Geometry check sheet. Reference: the model listing, model coordinates, mm. Face numbers are marked on the shaded views. A direction names the side the tool comes from. Give positions to 0.01 mm unless a question says otherwise; leave off trailing zeros. Write each loop counter-clockwise with the first axis right and the second up, starting at its lowest first coordinate (ties: lowest second). Pieces come first, ordered by that corner, then holes. Notation, with made-up numbers: (56, 2) - (61, 2) arc R18 cw to (61, 14) - close; hole circle Ø4 at (2, -21.5). An arc over 180 degrees is marked (long way). One line per question, with ' | ' between items. Start each with the question number.
Q1. Section check B-B on x = 0. Record the boundary of the cut face in (y, z).
Q2. Section check A-A on z = 0. Record the boundary of the cut face in (x, y), and give its area (3 significant figures).
Q3. Set-up check for the marked faces 4, 5 and 6: record each of +Z, -Z, +X, -X, +Y, -Y from which the full face is reachable in a straight line by a thin tool's end or side.
Q4. Thickness scan on L1, parallel to Y at x = 0.5, z = 0; L2, parallel to X at y = 53.5, z = 0; L3, parallel to Z at x = -0.25, y = 34.8. Record the ranges inside material, lowest first. Write a range as [from, to].
Q5. Section check C-C on y = 34.8. Record the boundary of the cut face in (x, z).
Q6. Section check D-D on x = 4. Record the boundary of the cut face in (y, z).
Q7. Release check for a two-part mould opening along X. For the marked faces 1, 2 and 3 record: +X half, -X half, draft (parallel to the pull), parting line (faces both ways), or undercut.
Q8. Gauge pin test, flat ends, axial feed: P1, Ø4, axis at y = 38, z = 4, coming from the -X side; P2, Ø2, axis at x = 4.5, z = 1, coming from the -Y side; P3, Ø1, axis at x = -1, z = -3.5, coming from the +Y side. Record the tip position at first contact, or that the pin passes through.
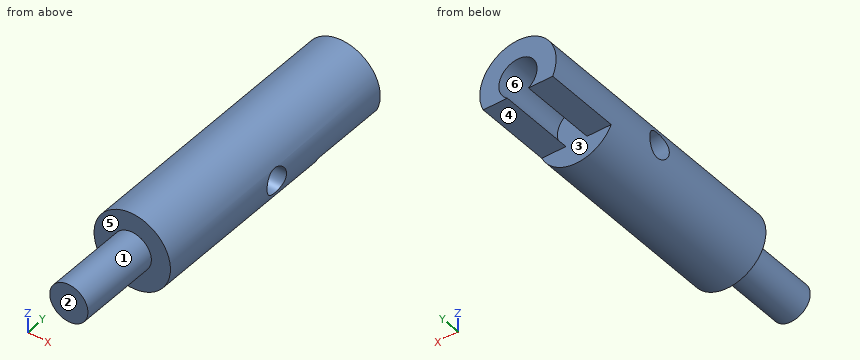
```python
from build123d import *

# Parameters (mm, degrees)
SKETCH_1_R               = 6
EXTRUDE_1_DEPTH          = 56
CUT_EXTRUDE_START        = -12
CUT_EXTRUDE_1_DEPTH      = 12
SKETCH_3_R               = 6
SKETCH_3_R_2             = 3
CUT_EXTRUDE_2_DEPTH      = 13
CUT_EXTRUDE_6_DEPTH      = 57.639209034
CUT_EXTRUDE_6_DEPTH_BACK = 57.639209034
SKETCH_6_R               = 2


with BuildPart() as part:
    # ｽｹｯﾁ1 → ﾎﾞｽ - 押し出し1 (new body)
    with BuildSketch(Plane(origin=(0, 0, 0), x_dir=(1, 0, 0), z_dir=(0, 1, 0))):
        with Locations(Location((0, 0, 0), (0, 0, 270))):
            Circle(SKETCH_1_R)
    extrude(amount=EXTRUDE_1_DEPTH)

    # ｽｹｯﾁ2 → ｶｯﾄ - 押し出し1 (cut)
    with BuildSketch(Plane(origin=(0, 56, 0), x_dir=(1, 0, 0), z_dir=(0, 1, 0)).offset(CUT_EXTRUDE_START)):
        with BuildLine():
            Line((1.658312395, 2.5), (5.454356057, 2.5))
            ThreePointArc((5.454356057, 2.5), (0, 6), (-5.454356057, 2.5))
            Line((-5.454356057, 2.5), (-1.658312395, 2.5))
            ThreePointArc((-1.658312395, 2.5), (0, -3), (1.658312395, 2.5))
        make_face()
    extrude(amount=CUT_EXTRUDE_1_DEPTH, mode=Mode.SUBTRACT)

    # ｽｹｯﾁ3 → ｶｯﾄ - 押し出し2 (cut)
    with BuildSketch(Plane.XZ):
        with Locations(Location((0, 0, 0), (0, 0, 270))):
            Circle(SKETCH_3_R)
        with Locations(Location((0, 0, 0), (0, 0, 270))):
            Circle(SKETCH_3_R_2, mode=Mode.SUBTRACT)
    extrude(amount=-CUT_EXTRUDE_2_DEPTH, mode=Mode.SUBTRACT)

    # ｽｹｯﾁ6 → ｶｯﾄ - 押し出し6 (cut, two sides: drawn at the far end of the back side and taken through both)
    with BuildSketch(Plane(origin=(0, 0, 0), x_dir=(0, 0, -1), z_dir=(1, 0, 0)).offset(-CUT_EXTRUDE_6_DEPTH_BACK)):
        with Locations((0, 34.8)):
            Circle(SKETCH_6_R)
    extrude(amount=CUT_EXTRUDE_6_DEPTH + CUT_EXTRUDE_6_DEPTH_BACK, mode=Mode.SUBTRACT)


solid = part.part
```
Working result:
1) outline: (0, -3) - (13, -3) - (13, -6) - (44, -6) - (44, 3) - (56, 3) - (56, 6) - (13, 6) - (13, 3) - (0, 3) - close; hole circle Ø4 at (34.8, 0)
2) outline: (-6, 13) - (-3, 13) - (-3, 0) - (3, 0) - (3, 13) - (6, 13) - (6, 32.8) - (-6, 32.8) - close; (-6, 36.8) - (6, 36.8) - (6, 56) - (3, 56) - (3, 44) - (-3, 44) - (-3, 56) - (-6, 56) - close | area: 474 mm2
3) face 4: -Z, +X, -X, +Y | face 5: -Y | face 6: +Y
4) L1: y = [0, 32.8], [36.8, 44] | L2: x = [-6, -3], [3, 6] | L3: z = [-5.99, -2], [2, 5.99]
5) outline: (-5.66, -2) arc R6 ccw to (5.66, -2) - close; (-5.66, 2) - (5.66, 2) arc R6 ccw to start
6) outline: (13, -4.47) - (44, -4.47) - (44, -2.5) - (56, -2.5) - (56, 4.47) - (13, 4.47) - close; hole circle Ø4 at (34.8, 0)
7) face 1: parting line | face 2: draft | face 3: undercut
8) P1: stops at x = -5.66 | P2: stops at y = 13 | P3: stops at y = 44
